Build history of the part. All positions in model axes, mm. Give positions to 0.01 mm unless a question says otherwise; leave off trailing zeros. Order: outer loops, then holes, each group sorted by start corner. A loop starts at its lowest first (then second) coordinate and runs counter-clockwise, first axis right, second up. Notation, with made-up numbers: M -5,3 L 17,3 A21 ccw 17,20 Z; hole C -5.75,29 d4. An arc over 180 degrees is marked long. One line per item, written item: value. Start each with the question number.
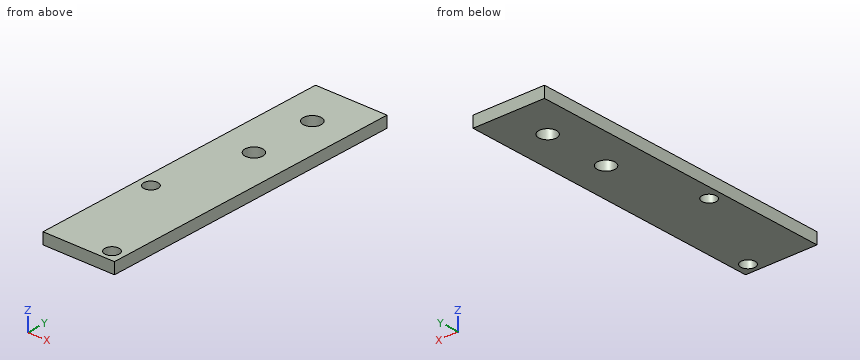
from build123d import *

# Parameters (mm, degrees)
SKETCH1_W           = 16.2
SKETCH1_H           = 70
BOSS_EXTRUDE1_DEPTH = 2.54
SKETCH4_R           = 1.6
CUT_EXTRUDE1_DEPTH  = 2.54
SKETCH6_R           = 2
CUT_EXTRUDE3_DEPTH  = 3.54


with BuildPart() as part:
    # Sketch1 → Boss-Extrude1 (new body)
    with BuildSketch(Plane.XY):
        with Locations((8.1, 35)):
            Rectangle(SKETCH1_W, SKETCH1_H)
    extrude(amount=BOSS_EXTRUDE1_DEPTH)

    # Sketch4 → Cut-Extrude1 (cut)
    with BuildSketch(Plane(origin=(0, 0, 0), x_dir=(-1, 0, 0), z_dir=(0, 0, -1))):
        with Locations((-13.4, 2.54)):
            Circle(SKETCH4_R)
        with Locations((-2.8, 24.54)):
            Circle(SKETCH4_R)
    extrude(amount=-CUT_EXTRUDE1_DEPTH, mode=Mode.SUBTRACT)

    # Sketch6 → Cut-Extrude3 (cut, through all)
    with BuildSketch(Plane.XY.offset(2.54)):
        with Locations((8.1, 60)):
            Circle(SKETCH6_R)
        with Locations((8.1, 45)):
            Circle(SKETCH6_R)
    extrude(amount=-CUT_EXTRUDE3_DEPTH, mode=Mode.SUBTRACT)


solid = part.part
1) Slice it at A-A (x = 8.1). List the corners of the cut face in (y, z), plus the area to 3 significant figures.
2) Drill centre lines: line 1 (Y direction, x = 8.1, z = 1.75); line 2 (Y direction, x = 7.5, z = 1.1); line 3 (Y direction, x = 2.75, z = 0.7). Where is each one in solid material? Low to high.
3) Slice it at B-B (x = 13.4). List the corners of the cut face in (y, z), plus the area to 3 significant figures.
4) Drop a flat-ended pin along its axis: P1, Ø1.9, axis at x = 2.8, y = 24.54, coming from the +Z side (3 decimals). Give the stop position or say it passes through.
5) Slice it at D-D (y = 24.54). List the corners of the cut face in (x, z), plus the area to 3 significant figures.
6) Slice it at C-C (z = 2). List the corners of the cut face in (x, y).
Results list:
1. outline: M 0,0 L 43,0 L 43,2.54 L 0,2.54 Z; M 47,0 L 58,0 L 58,2.54 L 47,2.54 Z; M 62,0 L 70,0 L 70,2.54 L 62,2.54 Z
1. area: 157 mm²
2. line 1: y = 0 to 43, 47 to 58, 62 to 70
2. line 2: y = 0 to 43.09, 46.91 to 58.09, 61.91 to 70
2. line 3: y = 0 to 22.94, 26.14 to 70
3. outline: M 0,0 L 0.94,0 L 0.94,2.54 L 0,2.54 Z; M 4.14,0 L 70,0 L 70,2.54 L 4.14,2.54 Z
3. area: 170 mm²
4. P1: passes through
5. outline: M 0,0 L 1.2,0 L 1.2,2.54 L 0,2.54 Z; M 4.4,0 L 16.2,0 L 16.2,2.54 L 4.4,2.54 Z
5. area: 33.0 mm²
6. outline: M 0,0 L 16.2,0 L 16.2,70 L 0,70 Z; hole C 2.8,24.54 d3.2; hole C 8.1,45 d4; hole C 8.1,60 d4; hole C 13.4,2.54 d3.2
